```python
from build123d import *

# Parameters (mm, degrees)
F0_W     = 290.903047
F0_H     = 114.028264
F0_R     = 22.227707
F1_DEPTH = 101.6
F3_DEPTH = 25.4


with BuildPart() as f1:
    # F0 (on Top) → F1 (new body)
    with BuildSketch(Plane.XY):
        with Locations((79.182141, -6.367212)):
            Rectangle(F0_W, F0_H)
        with Locations((-36.404692, -33.608936)):
            Circle(F0_R, mode=Mode.SUBTRACT)
    extrude(amount=F1_DEPTH)

    # F2 (on face) → F3 (cut)
    with BuildSketch(Plane.XY.offset(101.6)):
        with BuildLine():
            Line((113.667183, 17.614277), (90.719864, 17.614277))
            Line((90.719864, 17.614277), (90.719864, 3.507722))
            ThreePointArc((90.719864, 3.507722), (96.879223, -42.829117), (113.667183, 0.796618))
            Line((113.667183, 0.796618), (113.667183, 17.614277))
        make_face()
    extrude(amount=F3_DEPTH, mode=Mode.SUBTRACT)


solid = f1.part
```
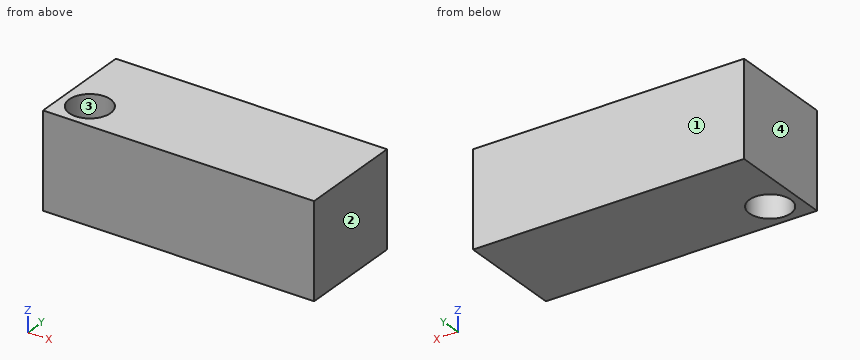
Work out the finished part from the listing and answer in its coordinate system (mm). Face numbers are marked on the shaded views. Coordinates: 2 decimals unless noted, no trailing zeros. Loops run counter-clockwise (first coordinate to the right, second up) from the corner with the lowest first, then second, coordinate; pieces in that order, holes last. Notation, with made-up numbers: (-38, 26.25) - (-29, 26.25) arc R27 ccw to (-29, 60.25) - close; hole circle Ø9 at (80.25, 26.25). An arc over 180 degrees is marked (long way). Use a Markdown table: item, result.
Item 1: The mould has two halves that part along X. Classify the marked faces 1, 2, 3 and 4: +X half, -X half, draft (parallel to the pull), parting line (faces both ways), or undercut.
Evaluation:
| item | result |
|---|---|
| face 1 | draft |
| face 2 | +X half |
| face 3 | undercut |
| face 4 | -X half |
Item 2: Consider probe 1 along Y at (x, z) = (-16, 30); probe 2 along X at (y, z) = (-43, 16); probe 3 along X at (y, z) = (-16.5, 22). Determine where each line is inside the solid, lowest interval first. Write a range as from..to.
Evaluation:
| item | result |
|---|---|
| probe 1 | y = -63.38..-42.42, -24.79..50.65 |
| probe 2 | x = -66.27..-56.55, -16.26..224.63 |
| probe 3 | x = -66.27..-50.59, -22.21..224.63 |
Item 3: Find section A-A, the plane y = -21. Determine the outline of the cut face in (x, z), and give its area (3 significant figures).
Evaluation:
| item | result |
|---|---|
| outline | (-66.27, 0) - (-54.71, 0) - (-54.71, 101.6) - (-66.27, 101.6) - close; (-18.1, 0) - (224.63, 0) - (224.63, 101.6) - (-18.1, 101.6) - close |
| area | 25,800 mm2 |
Item 4: Find section B-B, the plane z = 81.5. Determine the outline of the cut face in (x, y).
Evaluation:
| item | result |
|---|---|
| outline | (-66.27, -63.38) - (224.63, -63.38) - (224.63, 50.65) - (-66.27, 50.65) - close; hole circle Ø44.46 at (-36.4, -33.61) |
